Can you work these out from the model? Positions are in its coordinate system, mm. A direction names the side the tool comes from. Give positions to 0.01 mm unless a question says otherwise; leave off trailing zeros.
1. On a 3-axis mill with a long thin cutter (end or side, diameter ignored), from which of +Z, -Z, +X, -X, +Y, -Y can I reach the whole of each face in a straight line? I mean faces 5 (the conical face through (16.95, 2.15, 0.25)), 6 (the flat face through (9.39, 0.64, 5.72)). Say none if no direction works.
2. If I drill on probe 1 along X at (y, z) = (11, 1); probe 2 along Y at (x, z) = (8.25, 9.75); probe 3 along Y at (x, z) = (6.75, 3), over which ranges is the centre line in solid material (lowest first)?
3. Thinking about a two-plate mould opening in Y: for faces 1 (the conical face through (2.15, 2.1, 12.45)), 2 (the cylindrical face through (8.66, 13.4, 6.26)), 3 (the conical face through (16.9, 16.95, 0.25)), 4 (the flat face through (0, 9, 6)), which applies, pulls with the +Y half, pulls with the -Y half, needs draft (parallel to the pull), parting line crosses it, or undercut?
```python
from build123d import *

# Parameters (mm, degrees)
F0_W     = 19.05
F0_H     = 19.05
F1_DEPTH = 12.7
F3_DEPTH = 19.05
F6_R     = 3.96875
F7_DEPTH = 19.05


with BuildPart() as f1:
    # F0 (on Top) → F1 (new body)
    with BuildSketch(Plane.XY):
        with Locations((9.525, 9.525)):
            Rectangle(F0_W, F0_H)
    extrude(amount=F1_DEPTH)

    # F2 (on face) → F3 (cut)
    with BuildSketch(Plane(origin=(0, 0, 0), x_dir=(0, -1, 0), z_dir=(-1, 0, 0))):
        Polygon((0, 7.62), (-1.27, 6.35), (0, 5.08), align=None)
    extrude(amount=-F3_DEPTH, mode=Mode.SUBTRACT)

    # F6 (on face) → F7 (cut)
    with BuildSketch(Plane(origin=(0, 0, 0), x_dir=(1, 0, 0), z_dir=(0, 0, -1))):
        with Locations((9.525, -9.525)):
            Circle(F6_R)
    extrude(amount=-F7_DEPTH, mode=Mode.SUBTRACT)

    # F8 (on mid) + F5 (on mid) → F9 (revolve, cut)
    with BuildSketch(Plane(origin=(9.525, 0, 0), x_dir=(0, -1, 0), z_dir=(-1, 0, 0))):
        Polygon((-32.2430354842, 9.1649367963), (-19.05, 12.7), (-32.2430354842, 16.2350632037), align=None)
    with BuildSketch(Plane(origin=(9.525, 0, 0), x_dir=(0, -1, 0), z_dir=(-1, 0, 0))):
        Polygon((8.4822997993, 2.2728253812), (0, 0), (8.4822997993, 0), align=None)
    revolve(axis=Axis((9.525, 9.525, 12.7), (0, 0, -1)), mode=Mode.SUBTRACT)


solid = f1.part
```
Checks:
1. face 5: -Z, +X, -Y
1. face 6: +X, -X, -Y
2. probe 1: x = 0 to 5.84, 13.21 to 19.05
2. probe 2: y = 0 to 5.77, 13.28 to 19.05
2. probe 3: y = 0 to 6.69, 12.36 to 19.05
3. face 1: pulls with the -Y half
3. face 2: undercut
3. face 3: pulls with the +Y half
3. face 4: needs draft
